Here's how the part is built. I have some questions about the finished solid (model axes, mm). A direction names the side the tool comes from. Round coordinates to 2 decimals unless told otherwise and drop trailing zeros. Loops run counter-clockwise (first coordinate to the right, second up) from the corner with the lowest first, then second, coordinate; pieces in that order, holes last. Notation, with made-up numbers: M -28,-16.5 L -14,-16.5 A33 cw -14,14.5 Z; hole C 85.25,25 d7. An arc over 180 degrees is marked long. Use a Markdown table: item, result.
Autodesk Fusion 360 part; units mm, degrees
sketch "Sketch1" plane through (0, 0, 0) normal (0, 0, 1) x (1, 0, 0)
  line L0 (30, -40) -> (-30, -40)
  line L1 (-30, -40) -> (-30, 40)
  line L2 (-27, 40) -> (27, 40)
  line L3 (30, 40) -> (30, -40)
  line L4 (30, -40) -> (-30, 40) construction
  line L5 (-30, -40) -> (30, 40) construction
  line L6 (27, -37) -> (-27, -37)
  line L7 (-27, -37) -> (-27, 37)
  line L8 (-27, 37) -> (27, 37)
  line L9 (27, 37) -> (27, -37)
  line L10 (27, 37) -> (27, 40)
  line L11 (-27, 37) -> (-27, 40)
  line L12 (27, 40) -> (30, 40)
  line L13 (-30, 40) -> (-27, 40)
  line L14 (13.5, 17.5) -> (-13.5, 17.5)
  line L15 (-13.5, 17.5) -> (-13.5, -17.5)
  line L16 (-13.5, -17.5) -> (13.5, -17.5)
  line L17 (13.5, -17.5) -> (13.5, 17.5)
  line L18 (13.5, 17.5) -> (-13.5, -17.5) construction
  line L19 (-13.5, 17.5) -> (13.5, -17.5) construction
  line L20 (-13.5, -17.5) -> (13.5, -17.5)
  line L21 (13.5, -17.5) -> (13.5, -19.5)
  line L22 (13.5, -19.5) -> (-13.5, -19.5)
  line L23 (-13.5, -19.5) -> (-13.5, -17.5)
  line L24 (13.5, 17.5) -> (15.5, 17.5)
  line L25 (15.5, 17.5) -> (15.5, 9.5)
  line L26 (15.5, 9.5) -> (13.5, 9.5)
  line L27 (13.5, 9.5) -> (13.5, 17.5)
  line L28 (-13.5, 17.5) -> (-15.5, 17.5)
  line L29 (-15.5, 17.5) -> (-15.5, 9.5)
  line L30 (-15.5, 9.5) -> (-13.5, 9.5)
  line L31 (-13.5, 9.5) -> (-13.5, 17.5)
  line L32 (7.5, 18) -> (10.5, 18)
  line L33 (10.5, 18) -> (10.5, 20)
  line L34 (10.5, 20) -> (7.5, 20)
  line L35 (7.5, 20) -> (7.5, 18)
  line L36 (7.5, 18) -> (10.5, 20) construction
  line L37 (10.5, 18) -> (7.5, 20) construction
  line L38 (0, 10) -> (0, 29)
  line L39 (-7.5, 20) -> (-7.5, 18)
  line L40 (-10.5, 20) -> (-7.5, 20)
  line L41 (-7.5, 18) -> (-10.5, 18)
  line L42 (-7.5, 18) -> (-10.5, 20) construction
  line L43 (-10.5, 18) -> (-10.5, 20)
  line L44 (-10.5, 18) -> (-7.5, 20) construction
  point P0 (9, 19)
  point P1 (-9, 19)
  dimension "d1" = 60
  dimension "d2" = 80
  dimension "d8" = 27
  dimension "d9" = 35
  dimension "d10" = 2
  dimension "d11" = 2
  dimension "d12" = 8
  dimension "d13" = 2
  dimension "d14" = 8
  dimension "d24" = 3
  dimension "d25" = 2
extrude "Extrude1" add sketch "Sketch1" along normal blind 3 contours L6 L7 L8 L9 | L14 L15 L16 L17 L20 L27 L31 | L17 L24 L25 L26 L27 | L15 L28 L29 L30 L31 | L16 L20 L21 L22 L23 | L32 L33 L34 L35 | L39 L40 L41 L43
extrude "Extrude2" add sketch "Sketch1" along normal blind 20 contours L0 L1 L3 L6 L7 L9 L10 L11 L12 L13
extrude "Extrude3" add sketch "Sketch1" along normal blind 10 contours L17 L24 L25 L26 L27 | L15 L28 L29 L30 L31 | L16 L20 L21 L22 L23
ref_plane "WorkPlane1" through (14.5, 13.5, 7) normal (0, 0, 1) x (1, 0, 0)
sketch "Sketch2" plane through (0, 0, 7) normal (0, 0, 1) x (1, 0, 0)
  line L0 (15.5, 9.5) -> (13.5, 9.5)
  line L1 (15.5, 17.5) -> (15.5, 9.5)
  line L2 (13.5, 9.5) -> (13.5, 17.5)
  line L3 (13.5, 17.5) -> (15.5, 17.5)
  line L4 (-15.5, 17.5) -> (-15.5, 9.5)
  line L5 (-13.5, 9.5) -> (-13.5, 17.5)
  line L6 (-15.5, 9.5) -> (-13.5, 9.5)
  line L7 (-13.5, 17.5) -> (-15.5, 17.5)
  line L8 (-13.5, 9.5) -> (-13.5, 17.5)
  line L9 (-13.5, 17.5) -> (-15.5, 17.5)
  line L10 (-15.5, 17.5) -> (-15.5, 9.5)
  line L11 (-15.5, 9.5) -> (-13.5, 9.5)
  line L12 (-13.5, -17.5) -> (13.5, -17.5)
  line L13 (13.5, -19.5) -> (-13.5, -19.5)
  line L14 (13.5, -17.5) -> (13.5, -19.5)
  line L15 (-13.5, -19.5) -> (-13.5, -17.5)
  line L16 (15.5, 9.5) -> (11, 9.5)
  line L17 (11, 9.5) -> (11, 17.5)
  line L18 (11, 17.5) -> (15.5, 17.5)
  line L19 (15.5, 17.5) -> (15.5, 9.5)
  line L20 (-13.5, 9.5) -> (-11, 9.5)
  line L21 (-11, 9.5) -> (-11, 17.5)
  line L22 (-11, 17.5) -> (-13.5, 17.5)
  line L23 (-13.5, 17.5) -> (-13.5, 9.5)
  line L24 (13.5, -17.5) -> (-13.5, -17.5)
  line L25 (-13.5, -17.5) -> (-13.5, -15)
  line L26 (-13.5, -15) -> (13.5, -15)
  line L27 (13.5, -15) -> (13.5, -17.5)
  dimension "d18" = 4.5
  dimension "d19" = 8
  dimension "d20" = 2.5
  dimension "d21" = 8
  dimension "d22" = 27
  dimension "d23" = 2.5
loft "Loft1" add profiles "Sketch2" section 1 face at (-4.5, -18.1667, 10) section 2 contours L12 L24 L25 L26 L27 | L12 L13 L14 L15 L24
loft "Loft2" add profiles "Sketch2" section 1 face at (14.8333, 14.8333, 10) section 2 contours L0 L1 L2 L3 L16 L18 L19 | L2 L16 L17 L18
loft "Loft3" add profiles "Sketch2" section 1 face at (-14.1667, 12.1667, 10) section 2 contours L4 L5 L6 L7 L8 L9 L10 L11 L23 | L5 L8 L20 L21 L22 L23
extrude "Extrude4" add sketch "Sketch1" along normal blind 8 contours L32 L33 L34 L35 | L39 L40 L41 L43
Q1. We'd pull the mould along Y, two halves only. Please class faces 4 (the flat face through (-14, 17.5, 7)), 5 (the flat face through (-7.5, 19, 5)), 6 (the flat face through (0, -19.5, 6)): pulls with the +Y half, pulls with the -Y half, needs draft (parallel to the pull), parting line crosses it, or undercut.
Return value:
| item | result |
|---|---|
| face 4 | pulls with the +Y half |
| face 5 | needs draft |
| face 6 | undercut |
Q2. Imagine slicing it at A-A, the plane z = 5.75. Please give me the cut outline in (x, y).
Return value:
| item | result |
|---|---|
| outline | M -30,-40 L 30,-40 L 30,40 L 27,40 L 27,-37 L -27,-37 L -27,40 L -30,40 Z; M -15.5,9.5 L -13.5,9.5 L -13.5,17.5 L -15.5,17.5 Z; M -13.5,-19.5 L 13.5,-19.5 L 13.5,-17.5 L -13.5,-17.5 Z; M -10.5,18 L -7.5,18 L -7.5,20 L -10.5,20 Z; M 7.5,18 L 10.5,18 L 10.5,20 L 7.5,20 Z; M 13.5,9.5 L 15.5,9.5 L 15.5,17.5 L 13.5,17.5 Z |
Q3. Imagine slicing it at C-C, the plane x = -1. Please give me the cut outline in (y, z), then the cut area to 3 significant figures.
Return value:
| item | result |
|---|---|
| outline | M -40,0 L 37,0 L 37,3 L -17.5,3 L -17.5,7 L -15,7 L -17.5,10 L -19.5,10 L -19.5,3 L -37,3 L -37,20 L -40,20 Z |
| area | 300 mm^2 |
Q4. Will these pins go through, and if not, where does the flat tip stop? P1, Ø1.6, axis at x = 9.5, y = 19, coming from the +Z side; P2, Ø12, axis at x = -15.5, y = 21, coming from the -Z side; P3, Ø1.5, axis at x = 9, z = 6.5, coming from the +Y side; P4, Ø1.5, axis at x = -6.5, z = 15, coming from the +Y side.
Return value:
| item | result |
|---|---|
| P1 | stops at z = 8 |
| P2 | stops at z = 0 |
| P3 | stops at y = 20 |
| P4 | stops at y = -37 |
Q5. Imagine slicing it at B-B, the plane z = 14. Please give me the cut outline in (x, y).
Return value:
| item | result |
|---|---|
| outline | M -30,-40 L 30,-40 L 30,40 L 27,40 L 27,-37 L -27,-37 L -27,40 L -30,40 Z |
Q6. Imagine slicing it at D-D, the plane y = 7. Please give me the cut outline in (x, z).
Return value:
| item | result |
|---|---|
| outline | M -30,0 L 30,0 L 30,20 L 27,20 L 27,3 L -27,3 L -27,20 L -30,20 Z |
Q7. I need wall thicknesses on line 1 (X direction, y = -23.5, z = 14.75); line 2 (X direction, y = 12, z = 6.5); line 3 (Y direction, x = -9, z = 6). Which ranges of each line are inside material? Lowest first, please. Write a range as from..to.
Return value:
| item | result |
|---|---|
| line 1 | x = -30..-27, 27..30 |
| line 2 | x = -30..-27, -15.5..-13.5, 13.5..15.5, 27..30 |
| line 3 | y = -40..-37, -19.5..-17.5, 18..20 |
Q8. For faces 1 (the flat face through (14, 17.5, 7)), 2 (the flat face through (9, 18, 5)), 3 (the flat face through (0, 37, 1)), which set-ups out of +Z, -Z, +X, -X, +Y, -Y let a thin tool reach every point of the face, with its end or its side?
Return value:
| item | result |
|---|---|
| face 1 | +Z, +Y |
| face 2 | +Z |
| face 3 | +Z, -Z, +Y |
